```python
from build123d import *

# Parameters (mm, degrees)
SKETCH1_W                        = 127
SKETCH1_H                        = 152.4
BOSS_EXTRUDE1_DEPTH              = 12.7
SKETCH2_R                        = 14.2875
CUT_EXTRUDE1_DEPTH               = 166.587741092
FILLET1_R                        = 12.7
F_1_4_20_TAPPED_HOLE1_AT_2_COUNT = 2
F_1_4_20_TAPPED_HOLE1_AT_2_PITCH = 38.1
SKETCH5_W                        = 12.7
SKETCH5_H                        = 19.05
BOSS_EXTRUDE2_DEPTH              = 12.7
SKETCH6_R                        = 0.79375
CUT_EXTRUDE2_DEPTH               = 149.649688866
SKETCH7_W                        = 38.1
SKETCH7_H                        = 12.7
CUT_EXTRUDE3_DEPTH               = 149.649688866
FILLET2_START                    = -1
FILLET2_DEPTH                    = 15
FILLET2_2_DEPTH                  = 12.7


with BuildPart() as part:
    # Sketch1 → Boss-Extrude1 (new body)
    with BuildSketch(Plane.XY):
        with Locations((0, 76.2)):
            Rectangle(SKETCH1_W, SKETCH1_H)
    extrude(amount=BOSS_EXTRUDE1_DEPTH)

    # Sketch2 → Cut-Extrude1 (cut, through all)
    with BuildSketch(Plane.XY.offset(12.7)):
        with Locations((0, 95.25)):
            Circle(SKETCH2_R)
        with BuildLine():
            Line((31.75, 95.25), (31.75, 50.8))
            Line((31.75, 50.8), (63.5, 50.8))
            Line((63.5, 50.8), (63.5, 152.4))
            Line((63.5, 152.4), (-63.5, 152.4))
            Line((-63.5, 152.4), (-63.5, 50.8))
            Line((-63.5, 50.8), (-31.75, 50.8))
            Line((-31.75, 50.8), (-31.75, 95.25))
            ThreePointArc((-31.75, 95.25), (0, 127), (31.75, 95.25))
        make_face()
    extrude(amount=-CUT_EXTRUDE1_DEPTH, mode=Mode.SUBTRACT)

    # Fillet1
    fillet1_edges = [part.edges().sort_by_distance(p)[0] for p in [
        (-31.75, 50.8, 6.35),
        (31.75, 50.8, 6.35),
    ]]
    fillet(fillet1_edges, radius=FILLET1_R)

    # Sketch3 → 1/4-20 Tapped Hole1 (revolve, cut)
    with BuildSketch(Plane(origin=(63.5, 44.45, 6.35), x_dir=(0, 0, -1), z_dir=(0, 1, 0))):
        Polygon((0, 0), (0, 18.043816902), (2.5527, 16.51), (2.5527, 0), align=None)
    f_1_4_20_tapped_hole1 = revolve(axis=Axis((69.85, 44.45, 6.35), (-1, 0, 0)), mode=Mode.SUBTRACT)

    # 1/4-20 Tapped Hole1 at 2: 1/4-20 Tapped Hole1 ×2
    with Locations(*[(0, -i * F_1_4_20_TAPPED_HOLE1_AT_2_PITCH, 0) for i in range(1, F_1_4_20_TAPPED_HOLE1_AT_2_COUNT)]):
        add(f_1_4_20_tapped_hole1, mode=Mode.SUBTRACT)

    # Sketch5 → Boss-Extrude2 (add)
    with BuildSketch(Plane(origin=(63.5, 0, 0), x_dir=(0, 0, -1), z_dir=(1, 0, 0))):
        with Locations((-6.35, 25.4)):
            Rectangle(SKETCH5_W, SKETCH5_H)
    boss_extrude2 = extrude(amount=BOSS_EXTRUDE2_DEPTH)

    # Sketch6 → Cut-Extrude2 (cut, through all)
    with BuildSketch(Plane.XY.offset(12.7)):
        with Locations((63.5, 35.71875)):
            Circle(SKETCH6_R)
        with Locations((63.5, 15.08125)):
            Circle(SKETCH6_R)
    cut_extrude2 = extrude(amount=-CUT_EXTRUDE2_DEPTH, mode=Mode.SUBTRACT)

    # Mirror1: 1/4-20 Tapped Hole1, Boss-Extrude2, Cut-Extrude2 across plane
    add(f_1_4_20_tapped_hole1.mirror(Plane(origin=(0, 0, 0), x_dir=(0, 0, 1), z_dir=(1, 0, 0))), mode=Mode.SUBTRACT)
    add(boss_extrude2.mirror(Plane(origin=(0, 0, 0), x_dir=(0, 0, 1), z_dir=(1, 0, 0))))
    add(cut_extrude2.mirror(Plane(origin=(0, 0, 0), x_dir=(0, 0, 1), z_dir=(1, 0, 0))), mode=Mode.SUBTRACT)

    # Mirror1 copy 1 sketch → Mirror1 copy 1 (revolve, cut)
    with BuildSketch(Plane(origin=(-63.5, 6.35, 6.35), x_dir=(0, 0, -1), z_dir=(0, 1, 0))):
        Polygon((0, 0), (0, -18.043816902), (2.5527, -16.51), (2.5527, 0), align=None)
    revolve(axis=Axis((-69.85, 6.35, 6.35), (-1, 0, 0)), mode=Mode.SUBTRACT)

    # Sketch7 → Cut-Extrude3 (cut, through all)
    with BuildSketch(Plane.XY.offset(12.7)):
        with Locations((0, 6.35)):
            Rectangle(SKETCH7_W, SKETCH7_H)
    extrude(amount=-CUT_EXTRUDE3_DEPTH, mode=Mode.SUBTRACT)

    # Fillet2: read off the stored shape, not the designer's step
    # Fillet2 outline → Fillet2 (cut)
    with BuildSketch(Plane.XY.offset(FILLET2_START)):
        with BuildLine():
            Line((19.05, 0), (25.4, 0))
            ThreePointArc((25.4, 0), (20.909871939, 1.859871939), (19.05, 6.35))
            Line((19.05, 6.35), (19.05, 0))
        make_face()
        with BuildLine():
            Line((-19.05, 0), (-19.05, 6.35))
            ThreePointArc((-19.05, 6.35), (-20.909871939, 1.859871939), (-25.4, 0))
            Line((-25.4, 0), (-19.05, 0))
        make_face()
    extrude(amount=FILLET2_DEPTH, mode=Mode.SUBTRACT)

    # Fillet2 2 outline → Fillet2 2 (add)
    with BuildSketch(Plane.XY):
        with BuildLine():
            ThreePointArc((-19.05, 6.35), (-17.190128061, 10.840128061), (-12.7, 12.7))
            Line((-12.7, 12.7), (-19.05, 12.7))
            Line((-19.05, 12.7), (-19.05, 6.35))
        make_face()
        with BuildLine():
            ThreePointArc((12.7, 12.7), (17.190128061, 10.840128061), (19.05, 6.35))
            Line((19.05, 6.35), (19.05, 12.7))
            Line((19.05, 12.7), (12.7, 12.7))
        make_face()
    extrude(amount=FILLET2_2_DEPTH)


solid = part.part
```
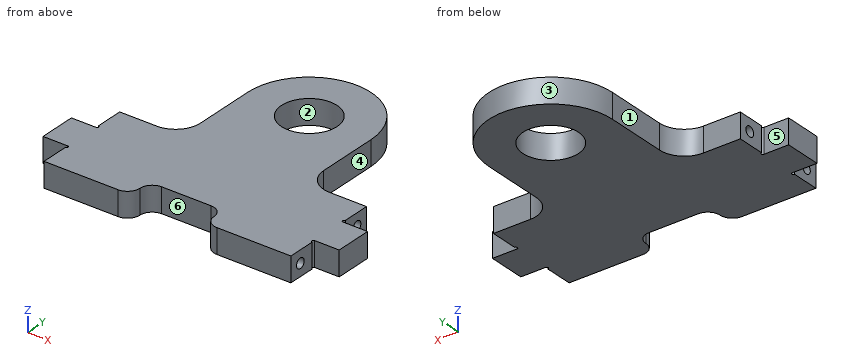
Work out the finished part from the listing and answer in its coordinate system (mm). Face numbers are marked on the shaded views. A direction names the side the tool comes from. Coordinates: 2 decimals unless noted, no trailing zeros. Loops run counter-clockwise (first coordinate to the right, second up) from the corner with the lowest first, then second, coordinate; pieces in that order, holes last. Notation, with made-up numbers: M 56.25,42 L 67.25,42 A11 cw 67.25,57 Z; hole C 81.25,27 d1. An arc over 180 degrees is marked long. Use CSV: the item, a comma, the result in double quotes. Start each with the question number.
(1) Consider line 1 (Y direction, x = 57.25, z = 6.35); line 2 (Z direction, x = 58, y = 44); line 3 (X direction, y = 66.5, z = 10.5). Determine where each line is inside the solid, lowest interval first.
(2) Find section C-C, the plane x = 17. Give the vertices of the cut face in (y, z), then the cut area to 3 significant figures.
(3) Find section A-A, the plane x = 0. Give the vertices of the cut face in (y, z), then the cut area to 3 significant figures.
(4) For the marked faces 4, 5 and 6, determine the directions among +Z, -Z, +X, -X, +Y, -Y from which every point of the face is accessible in a straight line to the end or side of a thin tool.
(5) Given pin 1 Ø4 at (y, z) = (9, 6.5) entering from +X; pin 2 Ø4 at (x, z) = (-54.5, 5.5) entering from +Y; pin 3 Ø3 at (x, z) = (-12.5, 9.5) entering from -Y, each flat-ended and moving along its own axis, determine where each tip first touches the part or whether it passes through.
(6) Find section B-B, the plane y = 49. Give the vertices of the cut face in (x, z), then the cut area to 3 significant figures.
(7) For a pull along Y with two mould halves and no side action, classify the marked faces 1, 2 and 3 as +Y half, -Y half, draft (parallel to the pull), parting line (faces both ways), or undercut.
Recorded:
1,line 1,"y = 0 to 3.8, 8.9 to 41.9, 47 to 50.8"
1,line 2,"z = 0 to 3.84, 8.86 to 12.7"
1,line 3,"x = -31.75 to 31.75"
2,outline,"M 11.02,0 L 122.07,0 L 122.07,12.7 L 11.02,12.7 Z"
2,area,"1,410 mm^2"
3,outline,"M 12.7,0 L 80.96,0 L 80.96,12.7 L 12.7,12.7 Z; M 109.54,0 L 127,0 L 127,12.7 L 109.54,12.7 Z"
3,area,"1,090 mm^2"
4,face 4,"+Z, -Z, +X, +Y"
4,face 5,"+Z, -Z, -X, +Y"
4,face 6,"+Z, -Z, -Y"
5,pin 1,"stops at x = 63.5"
5,pin 2,"stops at y = 50.8"
5,pin 3,"stops at y = 12.57"
6,outline,"M -63.5,0 L 63.5,0 L 63.5,12.7 L -63.5,12.7 Z"
6,area,"1,610 mm^2"
7,face 1,"draft"
7,face 2,"undercut"
7,face 3,"+Y half"
